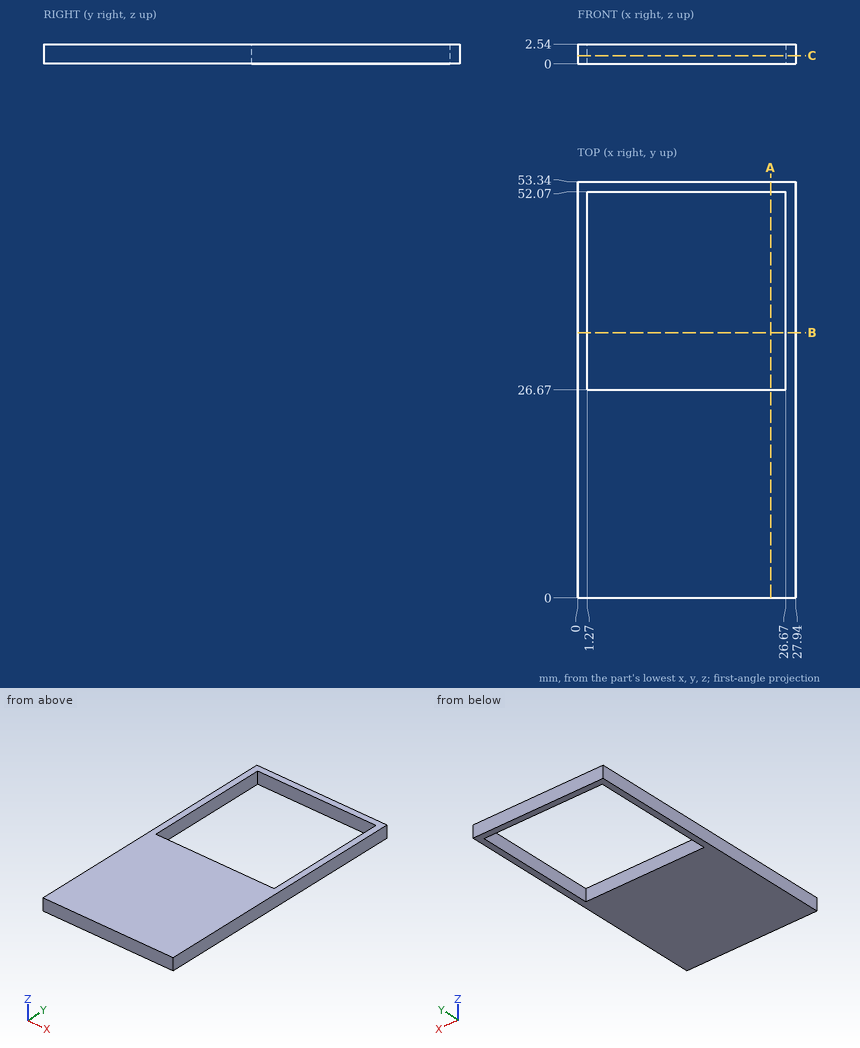
Source: three-view drawing plus pictorial views. Frame: mm from the lowest corner of the part. Give positions to 0.01 mm unless a question says otherwise; leave off trailing zeros. Order: outer loops, then holes, each group sorted by start corner. A loop starts at its lowest first (then second) coordinate and runs counter-clockwise, first axis right, second up. Notation, with made-up numbers: (-31, -26) -> (-4, -26) arc R22 cw to (-4, -18) -> close; hole circle Ø7 at (11, 60.25). An arc over 180 degrees is marked (long way). Write each question's results on one line, items separated by ' | '. Start each with the question number.
Item 1: Cut plane A-A on x = 24.75. Return the cut outline in (y, z).
Item 2: Cut plane C-C on z = 1.05. Return the cut outline in (x, y), then the cut area to 3 significant figures.
Item 3: Cut plane B-B on y = 34. Return the cut outline in (x, z), then the cut area to 3 significant figures.
Item 4: Line query: line 1 (Y direction, x = 9.5, z = 1.6); line 2 (X direction, y = 51.5, z = 1.7). Output: solid intervals per line, ascending.
Established:
1) outline: (0, 0) -> (26.67, 0) -> (26.67, 2.54) -> (0, 2.54) -> close; (52.07, 0) -> (53.34, 0) -> (53.34, 2.54) -> (52.07, 2.54) -> close
2) outline: (0, 0) -> (27.94, 0) -> (27.94, 53.34) -> (0, 53.34) -> close; hole (1.27, 26.67) -> (26.67, 26.67) -> (26.67, 52.07) -> (1.27, 52.07) -> close | area: 845 mm^2
3) outline: (0, 0) -> (1.27, 0) -> (1.27, 2.54) -> (0, 2.54) -> close; (26.67, 0) -> (27.94, 0) -> (27.94, 2.54) -> (26.67, 2.54) -> close | area: 6.45 mm^2
4) line 1: 0 to 26.67, 52.07 to 53.34 | line 2: 0 to 1.27, 26.67 to 27.94
